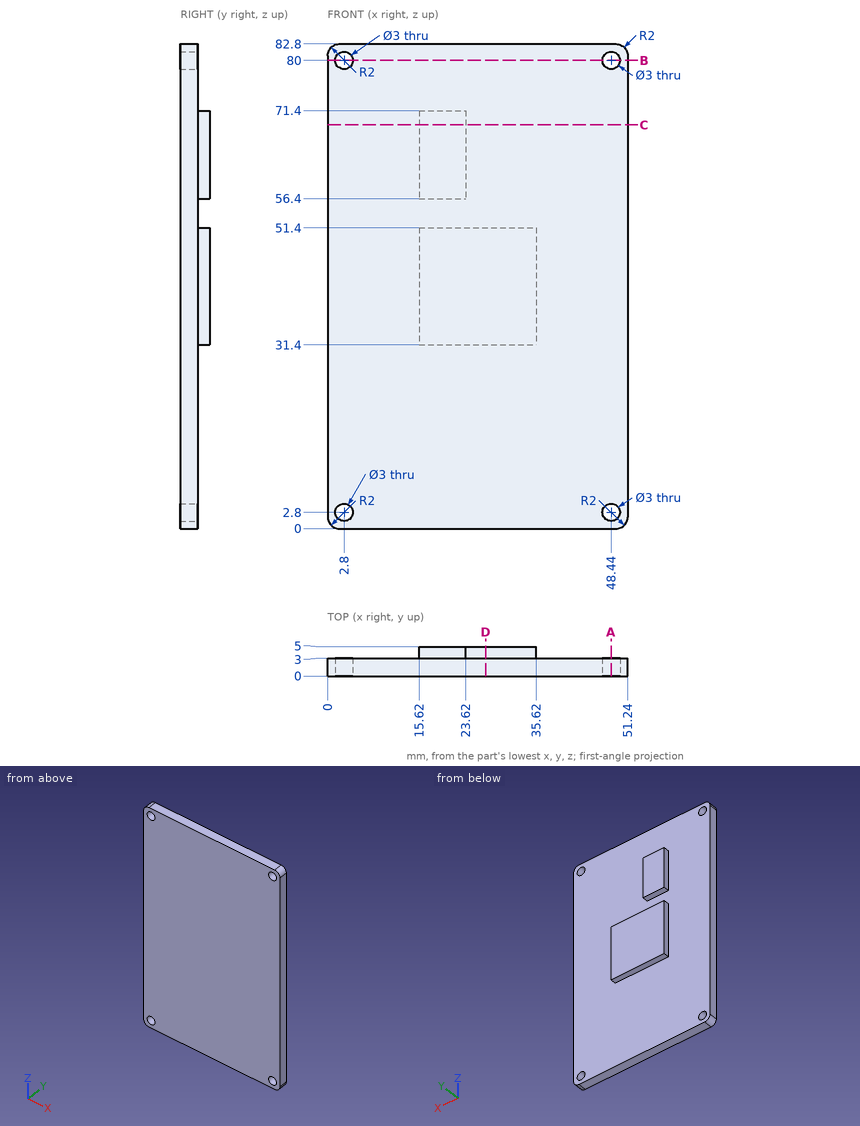
Answer from the drawing. Dimensions are ordinates in mm from the lowest x, y and z of the part. Coordinates: 2 decimals unless noted, no trailing zeros. Order: outer loops, then holes, each group sorted by start corner. A loop starts at its lowest first (then second) coordinate and runs counter-clockwise, first axis right, second up. Notation, with made-up numbers: M 0,50 L 53,50 A20 cw 53,80 Z; hole C -28,83.25 d2. An arc over 180 degrees is marked long. Put each result on its own line as item: value. Start each with the question number.
Item 1: Section C-C, the plane z = 69 is taken. Determine the outline of the cut face in (x, y), plus the area to 3 significant figures.
Item 2: Section B-B, the plane z = 80 is taken. Determine the outline of the cut face in (x, y), plus the area to 3 significant figures.
Item 3: Section A-A, the plane x = 48.44 is taken. Determine the outline of the cut face in (y, z), plus the area to 3 significant figures.
Item 4: Section D-D, the plane x = 27 is taken. Determine the outline of the cut face in (y, z).
Item 5: Consider probe 1 along X at (y, z) = (1.6, 2.8); probe 2 along Y at (x, z) = (11, 10.5); probe 3 along X at (y, z) = (3.05, 64.5). Determine where each line is inside the solid, lowest interval first. Write a range as [from, to].
Item 6: Given pin 1 Ø2 at (y, z) = (3.5, 64) entering from +X; pin 2 Ø4 at (x, z) = (48.44, 2.8) entering from +Y; pin 3 Ø0.6 at (x, y) = (27, 3.5) entering from +Z; pin 4 Ø1.6 at (y, z) = (4, 65) entering from -X, each flat-ended and moving along its own axis, determine where each tip first touches the part or whether it passes through.
Computed:
1. outline: M 0,0 L 51.24,0 L 51.24,3 L 23.62,3 L 23.62,5 L 15.62,5 L 15.62,3 L 0,3 Z
1. area: 170 mm2
2. outline: M 0,0 L 1.3,0 L 1.3,3 L 0,3 Z; M 4.3,0 L 46.94,0 L 46.94,3 L 4.3,3 Z; M 49.94,0 L 51.24,0 L 51.24,3 L 49.94,3 Z
2. area: 136 mm2
3. outline: M 0,0 L 3,0 L 3,1.3 L 0,1.3 Z; M 0,4.3 L 3,4.3 L 3,78.5 L 0,78.5 Z; M 0,81.5 L 3,81.5 L 3,82.8 L 0,82.8 Z
3. area: 230 mm2
4. outline: M 0,0 L 3,0 L 3,31.4 L 5,31.4 L 5,51.4 L 3,51.4 L 3,82.8 L 0,82.8 Z
5. probe 1: x = [0, 1.3], [4.3, 46.94], [49.94, 51.24]
5. probe 2: y = [0, 3]
5. probe 3: x = [15.62, 23.62]
6. pin 1: stops at x = 51.24
6. pin 2: stops at y = 3
6. pin 3: stops at z = 51.4
6. pin 4: stops at x = 15.62
